Verification items for the finished model (mm, model axes). Face numbers are marked on the shaded views. A direction names the side the tool comes from. Coordinates: 2 decimals unless noted, no trailing zeros. Order: outer loops, then holes, each group sorted by start corner. A loop starts at its lowest first (then second) coordinate and runs counter-clockwise, first axis right, second up. Notation, with made-up numbers: M 37.25,-9 L 80.25,-9 A35 cw 80.25,24 Z; hole C -26,5 d9. An arc over 180 degrees is marked long. Return JSON: item names as keys, results as strings.
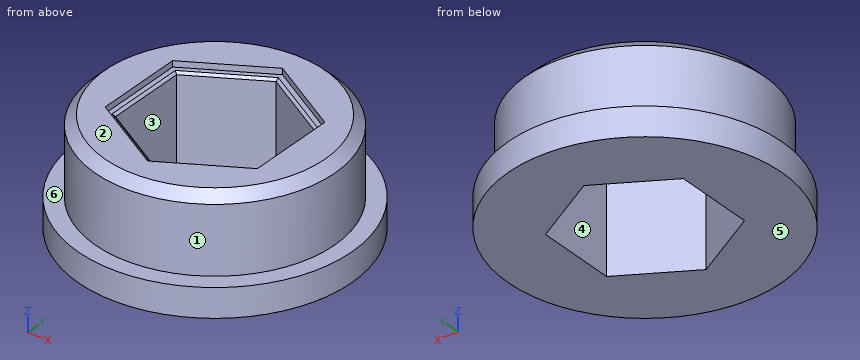
```python
from build123d import *

# Parameters (mm, degrees)
POCKET023_DEPTH = 22.001
POCKET024_DEPTH = 1.25
CHAMFER_SIZE    = 2
CHAMFER001_SIZE = 0.5


with BuildPart() as part:
    # Sketch032 (on XZ_Plane051 of Origin102) → Revolution010 (revolve)
    with BuildSketch(Plane.XZ):
        Polygon((0, 0), (28.5, 0), (28.5, 6), (24.95, 6), (24.95, 22), (0, 22), align=None)
    revolve(axis=Axis((0, 0, 0), (0, 0, 1)))

    # Sketch033 (on XY_Plane051 of Origin102) → Pocket023 (cut, through all)
    with BuildSketch(Plane.XY):
        Polygon((14.3875, 8.306627), (0, 16.613254), (-14.3875, 8.306627), (-14.3875, -8.306627), (0, -16.613254), (14.3875, -8.306627), align=None)
    extrude(amount=POCKET023_DEPTH, mode=Mode.SUBTRACT)

    # Sketch034 (on XY_Plane051 of Origin102) → Pocket024 (cut)
    with BuildSketch(Plane.XY.offset(22)):
        Polygon((15.875, -9.165436), (15.875, 9.165436), (0, 18.330871), (-15.875, 9.165436), (-15.875, -9.165436), (0, -18.330871), align=None)
    extrude(amount=-POCKET024_DEPTH, mode=Mode.SUBTRACT)

    # Chamfer
    chamfer_edges = [part.edges().sort_by_distance(p)[0] for p in [
        (-24.95, 0, 22),
    ]]
    chamfer(chamfer_edges, length=CHAMFER_SIZE)

    # Chamfer001
    chamfer001_edges = [part.edges().sort_by_distance(p)[0] for p in [
        (-14.3875, 0, 20.75),
        (-7.19375, 12.45994, 20.75),
        (7.19375, 12.45994, 20.75),
        (14.3875, 0, 20.75),
        (7.19375, -12.45994, 20.75),
        (-7.19375, -12.45994, 20.75),
    ]]
    chamfer(chamfer001_edges, length=CHAMFER001_SIZE)


with BuildPart() as part_1:
    # Body055 placement: moved
    add(part.part.moved(Location((-60, 60, 0))))


solid = part_1.part
```
Q1. Tool access check on the marked faces 4, 5 and 6. Record the directions out of +Z, -Z, +X, -X, +Y, -Y that give a thin tool (end or side, any length) a straight path to the whole face; none if there is none.
Values:
{"face 4": "+Z, -Z", "face 5": "-Z, +X, -X, +Y, -Y", "face 6": "+Z"}
Q2. Cross-section at B-B, the plane z = 14.25. Record the boundary of the cut face in (x, y), and give its area (3 significant figures).
Values:
{"outline": "C -60,60 d49.9; hole M -74.39,51.69 L -60,43.39 L -45.61,51.69 L -45.61,68.31 L -60,76.61 L -74.39,68.31 Z", "area": "1,240 mm^2"}
Q3. Go/stop test with flat-tipped pins: pin 1 (2 mm diameter, centred on x = -82.5, z = 19.5, fed in from -Y); pin 2 (2 mm diameter, centred on x = -77, z = 12, fed in from +Y); pin 3 (3 mm diameter, centred on x = -70.5, y = 68.5, fed in from -Z); pin 4 (8.5 mm diameter, centred on y = 61, z = 12.5, fed in from +X). Record where each tip stops, or that it passes through.
Values:
{"pin 1": "y = 47.34", "pin 2": "y = 79.14", "pin 3": "through", "pin 4": "x = -35.05"}
Q4. Material ranges on line 1 along Y through (x, z) = (-69, 2.75); line 2 along X through (y, z) = (51, 5.75); line 3 along Y through (x, z) = (-70, 15.75), recorded low to high.
Values:
{"line 1": "32.96 to 48.58, 71.42 to 87.04", "line 2": "-87.04 to -73.19, -46.81 to -32.96", "line 3": "37.14 to 49.16, 70.84 to 82.86"}
Q5. Draft check along Y on the marked faces 1, 2 and 3. Enter one of: pulls with the +Y half, pulls with the -Y half, needs draft (parallel to the pull), parting line crosses it, or undercut.
Values:
{"face 1": "parting line crosses it", "face 2": "needs draft", "face 3": "undercut"}
